Drawing for the job (mm, zero at the part's lowest x, y, z). A direction names the side the tool comes from. Round coordinates to 2 decimals unless told otherwise and drop trailing zeros. Write each loop counter-clockwise with the first axis right and the second up, starting at its lowest first coordinate (ties: lowest second). Pieces come first, ordered by that corner, then holes.
Item 1: Drop flat-ended pins along their axis: pin 1 Ø5 at (x, z) = (38, 99.5) entering from +Y; pin 2 Ø4 at (x, z) = (57.5, 190) entering from +Y; pin 3 Ø5 at (x, z) = (56.5, 180) entering from -Y. Give the stop position or say it passes through.
Item 2: 3-axis set-ups, long thin cutter, end or side, ignore diameter. For the marked faces 1, 2 and 3: which of +Z, -Z, +X, -X, +Y, -Y reach the whole face in a straight line?
Item 3: Band-saw the part on C-C, the plane z = 81. Write the cut outline in (x, y), then the cut area to 3 significant figures.
Item 4: Band-saw the part on D-D, the plane y = 30. Write the cut outline in (x, z), then the cut area to 3 significant figures.
Item 5: Wall check: probe 1 along Z at (x, y) = (14.5, 44.5); probe 2 along Z at (x, y) = (97, 21); probe 3 along X at (y, z) = (59, 111.5). Give the ranges that are in metal, low to high.
Item 6: Band-saw the part on A-A, the plane x = 55. Write the cut outline in (y, z).
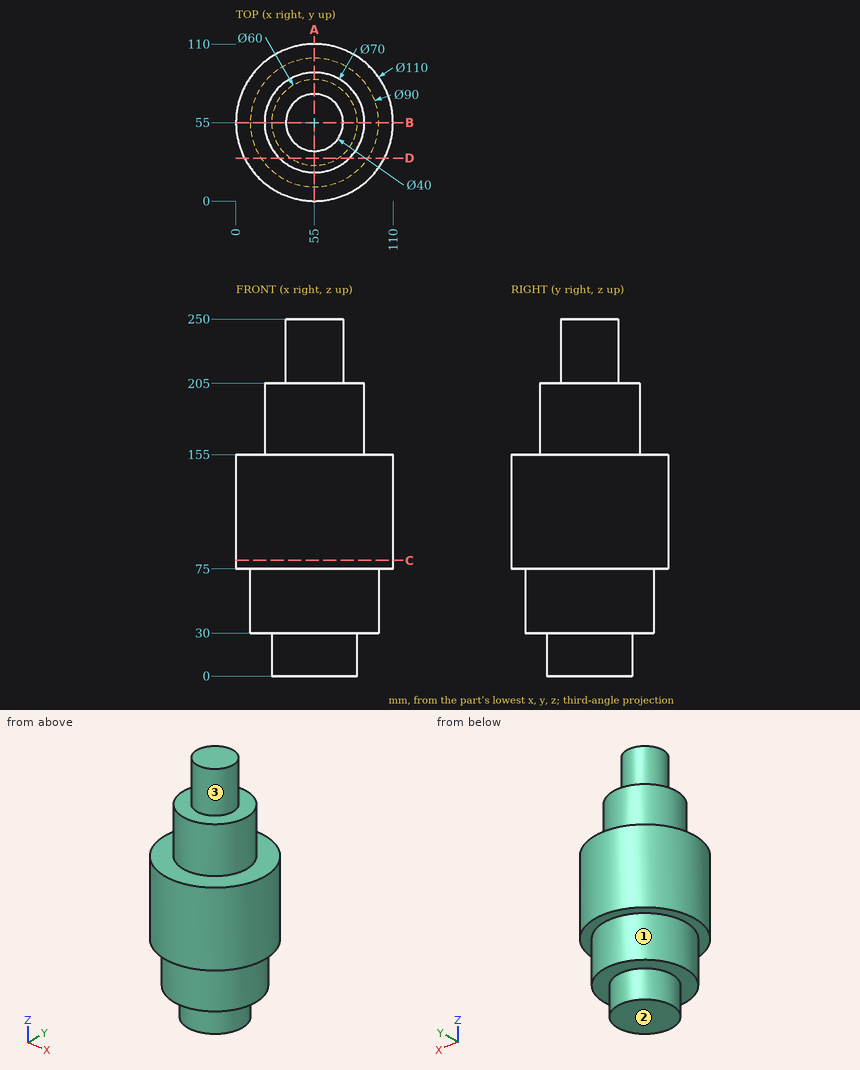
Results:
1. pin 1: stops at y = 108.05
1. pin 2: stops at y = 90
1. pin 3: stops at y = 20
2. face 1: -Z
2. face 2: -Z, +X, -X, +Y, -Y
2. face 3: +Z
3. outline: circle Ø110 at (55, 55)
3. area: 9,500 mm2
4. outline: (6.01, 75) - (17.58, 75) - (17.58, 30) - (38.42, 30) - (38.42, 0) - (71.58, 0) - (71.58, 30) - (92.42, 30) - (92.42, 75) - (103.99, 75) - (103.99, 155) - (79.49, 155) - (79.49, 205) - (30.51, 205) - (30.51, 155) - (6.01, 155) - close
4. area: 14,700 mm2
5. probe 1: z = 30 to 155
5. probe 2: z = 75 to 155
5. probe 3: x = 0.15 to 109.85
6. outline: (0, 75) - (10, 75) - (10, 30) - (25, 30) - (25, 0) - (85, 0) - (85, 30) - (100, 30) - (100, 75) - (110, 75) - (110, 155) - (90, 155) - (90, 205) - (75, 205) - (75, 250) - (35, 250) - (35, 205) - (20, 205) - (20, 155) - (0, 155) - close
